Input: part model. Units: mm. Frame: model coordinates. Face numbers are marked on the shaded views. A direction names the side the tool comes from. Coordinates: 2 decimals unless noted, no trailing zeros. Loops run counter-clockwise (first coordinate to the right, second up) from the corner with the lowest first, then second, coordinate; pieces in that order, holes last.
(1) Section A-A, the plane z = -15.5. Return loops of the section in (x, y), then the cut area to 3 significant figures.
(2) Set-up query: the marked faces 1, 2, 3, 4 and 5. Return all of +Z, -Z, +X, -X, +Y, -Y with unobstructed straight access to the full face (end or side cutting, diameter ignored); none if empty.
(3) Section B-B, the plane x = 10. Return loops of the section in (y, z).
(4) Line query: L1, parallel to Y at x = 9.25, z = -7.5; L2, parallel to Z at x = 16, y = -0.5; L3, parallel to Z at x = 4, y = 30.5. Output: solid intervals per line, ascending.
(5) Section D-D, the plane x = 16. Return loops of the section in (y, z), then the cut area to 3 significant figures.
(6) Mould query, pull axis Y, two halves, no side actions, for the marked faces 6, 7 and 8. Classes: released by +Y, released by -Y, zero draft, split by the parting line, or undercut.
(7) Contact query for flat-ended pins moving along their axis: P1, Ø7, axis at x = 12, z = -2.5, coming from the -Y side; P2, Ø6.5, axis at x = 10, y = -31, coming from the -Z side; P3, Ø5, axis at x = 9.5, y = 33, coming from the +Z side. Output: stop coordinate, or through.
(8) Section C-C, the plane z = -1. Return loops of the section in (x, y), then the cut area to 3 significant figures.
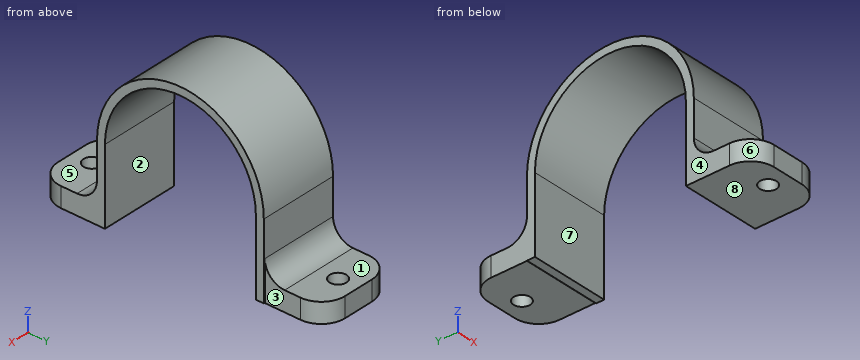
```python
from build123d import *

# Parameters (mm, degrees)
PAD001_DEPTH    = 20
POCKET_DEPTH    = 20
SKETCH003_W     = 5
SKETCH003_H     = 20
PAD002_DEPTH    = 15
SKETCH004_W     = 5
SKETCH004_H     = 19.712328
PAD003_DEPTH    = 15
FILLET_R        = 5
FILLET001_R     = 5
SKETCH005_R     = 2.1
POCKET001_DEPTH = 7
FILLET002_R     = 6


with BuildPart() as part:
    # Sketch001 → Pad001 (new body)
    with BuildSketch(Plane.YZ):
        with BuildLine():
            ThreePointArc((21, 0), (0, 21), (-21, 0))
            Line((-21, 0), (-21, -19))
            Line((21, -19), (-21, -19))
            Line((21, 0), (21, -19))
        make_face()
    extrude(amount=PAD001_DEPTH)

    # Sketch002 (on Face5 of Pad001) → Pocket (cut)
    with BuildSketch(Plane(origin=(0, 0, 0), x_dir=(0, 1, 0), z_dir=(-1, 0, 0))):
        with BuildLine():
            ThreePointArc((-19, 0), (0, -19), (19, 0))
            Line((19, 0), (19, 19))
            Line((-19, 19), (19, 19))
            Line((-19, 0), (-19, 19))
        make_face()
    extrude(amount=-POCKET_DEPTH, mode=Mode.SUBTRACT)

    # Sketch003 (on Face3 of Pocket) → Pad002 (join)
    with BuildSketch(Plane(origin=(0, -21, 0), x_dir=(0, 0, -1), z_dir=(0, -1, 0))):
        with Locations((16.5, 10)):
            Rectangle(SKETCH003_W, SKETCH003_H)
    extrude(amount=PAD002_DEPTH)

    # Sketch004 (on Face2 of Pad002) → Pad003 (join)
    with BuildSketch(Plane.ZX.offset(21)):
        with Locations((-16.558334, 9.856164)):
            Rectangle(SKETCH004_W, SKETCH004_H)
    extrude(amount=PAD003_DEPTH)

    # Fillet
    fillet_edges = [part.edges().sort_by_distance(p)[0] for p in [
        (9.856164, 21, -14.058334),
    ]]
    fillet(fillet_edges, radius=FILLET_R)

    # Fillet001
    fillet001_edges = [part.edges().sort_by_distance(p)[0] for p in [
        (10, -21, -14),
    ]]
    fillet(fillet001_edges, radius=FILLET001_R)

    # Sketch005 (on Face14 of Fillet001) → Pocket001 (cut)
    with BuildSketch(Plane(origin=(0, 0, -14), x_dir=(0, -1, 0), z_dir=(0, 0, 1))):
        with Locations((30.997393, 10)):
            Circle(SKETCH005_R)
        with Locations((-30.985943, 10)):
            Circle(SKETCH005_R)
    extrude(amount=-POCKET001_DEPTH, mode=Mode.SUBTRACT)

    # Fillet002
    fillet002_edges = [part.edges().sort_by_distance(p)[0] for p in [
        (0, 36, -16.558334),
        (19.712328, 36, -16.558334),
        (0, -36, -16.5),
        (20, -36, -16.5),
    ]]
    fillet(fillet002_edges, radius=FILLET002_R)


solid = part.part
```
Report:
1. outline: (0, -30) arc R6 ccw to (6, -36) - (14, -36) arc R6 ccw to (20, -30) - (20, -19) - (0, -19) - close; (0, 19) - (20, 19) - (20, 21) - (19.71, 21) - (19.71, 30) arc R6 ccw to (13.71, 36) - (6, 36) arc R6 ccw to (0, 30) - close; hole circle Ø4.2 at (10, -31); hole circle Ø4.2 at (10, 30.99)
1. area: 617 mm2
2. face 1: +Z, +X, -X, +Y
2. face 2: -Z, +X, -X
2. face 3: +Z, -Z, +X, +Y
2. face 4: +Z, -Z, -X, +Y, -Y
2. face 5: +Z, +X, -X, -Y
3. outline: (-36, -19) - (-33.1, -19) - (-33.1, -14) - (-36, -14) - close; (-28.9, -19) - (-19, -19) - (-19, 0) arc R19 cw to (19, 0) - (19, -19) - (21, -19) - (21, -19.06) - (28.89, -19.06) - (28.89, -14.06) - (26, -14.06) arc R5 cw to (21, -9.06) - (21, 0) arc R21 ccw to (-21, 0) - (-21, -9) arc R5 cw to (-26, -14) - (-28.9, -14) - close; (33.09, -19.06) - (36, -19.06) - (36, -14.06) - (33.09, -14.06) - close
4. L1: y = -21 to -19, 19 to 21
4. L2: z = 18.99 to 20.99
4. L3: z = -19.06 to -14.06
5. outline: (-35.66, -19) - (-19, -19) - (-19, 0) arc R19 cw to (19, 0) - (19, -19) - (21, -19) - (21, -19.06) - (35.55, -19.06) - (35.55, -14.06) - (26, -14.06) arc R5 cw to (21, -9.06) - (21, 0) arc R21 ccw to (-21, 0) - (-21, -9) arc R5 cw to (-26, -14) - (-35.66, -14) - close
5. area: 358 mm2
6. face 6: released by -Y
6. face 7: undercut
6. face 8: zero draft
7. P1: stops at y = -21
7. P2: stops at z = -19
7. P3: stops at z = -14.06
8. outline: (0, -21) - (20, -21) - (20, -19) - (0, -19) - close; (0, 19) - (20, 19) - (20, 21) - (0, 21) - close
8. area: 80.0 mm2
